Could you check a few things on this model? Use its own coordinates, in mm. A direction names the side the tool comes from. Give positions to 0.01 mm unless a question says otherwise; leave off trailing zeros. Loops run counter-clockwise (first coordinate to the right, second up) from the corner with the lowest first, then second, coordinate; pieces in that order, holes last. Notation, with made-up numbers: M -6,-12 L 37,-12 A5 cw 37,-5 Z; hole C 36,75 d10. An arc over 180 degrees is marked long. Return JSON: item names as keys, results as strings. Group by question number.
1. For pin 1 (2.5 mm diameter, centred on x = 2, y = 23.5, fed in from -Z); pin 2 (2.5 mm diameter, centred on x = 2.5, z = -56, fed in from -Y); pin 3 (5 mm diameter, centred on y = 24.5, z = -56, fed in from +X); pin 4 (5.5 mm diameter, centred on x = 2, z = -57.5, fed in from +Y), each with a flat end and sliding along its axis, tell me the tip position at first contact or that it passes through.
2. If we mould it in two halves opening along Y, with no side actions, what happens to faces 5 (the flat face through (3, -25, -52)), 6 (the flat face through (3, -20, -57)), 7 (the cylindrical face through (0.07, -0.243, 47.953)), 8 (the flat face through (0, 11.05, 60))? For each: +Y half, -Y half, draft (parallel to the pull), parting line (faces both ways), or undercut.
3. If we section it at C-C (y = 21.5): Write out the boundary of the cut face in (x, z), plus the area to 3 significant figures.
4. For faces 1 (the flat face through (3, 0, -52)), 2 (the flat face through (-1, 0, -62)), 3 (the flat face through (3, 25, -52)), 4 (the flat face through (0, -25, -57)), which set-ups out of +Z, -Z, +X, -X, +Y, -Y let a thin tool reach every point of the face, with its end or its side?
5. Please list where these lines run through material, in increasing order: line 1 (Z direction, x = 1, y = -23); line 2 (Y direction, x = -1, z = 51.5); line 3 (Z direction, x = 2.5, y = 0).
6. If we section it at B-B (z = 54.5): Write out the boundary of the cut face in (x, y).
7. If we section it at D-D (x = 3.75): Write out the boundary of the cut face in (y, z), plus the area to 3 significant figures.
8. If we section it at A-A (x = -3): Write out the boundary of the cut face in (y, z), plus the area to 3 significant figures.
```python
from build123d import *

# Parameters (mm, degrees)
F0_W     = 10
F0_H     = 124
F1_DEPTH = 30
F3_DEPTH = 10
F4_W     = 10
F4_H     = 10
F5_DEPTH = 5


with BuildPart() as f1:
    # F0 (on Front) → F1 (new body, symmetric)
    with BuildSketch(Plane.XZ):
        Rectangle(F0_W, F0_H)
    extrude(amount=F1_DEPTH, both=True)

    # F2 (on face) → F3 (cut)
    with BuildSketch(Plane.YZ.offset(5)):
        with BuildLine():
            Line((-11.05, 62), (-11.05, 59))
            ThreePointArc((-11.05, 59), (0, 47.95), (11.05, 59))
            Line((11.05, 59), (11.05, 62))
            Line((11.05, 62), (-11.05, 62))
        make_face()
    extrude(amount=-F3_DEPTH, mode=Mode.SUBTRACT)

    # F4 (on face) → F5 (cut)
    with BuildSketch(Plane.YZ.offset(5)):
        with Locations((-25, -57)):
            Rectangle(F4_W, F4_H)
        with Locations((25, -57)):
            Rectangle(F4_W, F4_H)
        with Locations((0, -57)):
            Rectangle(F4_W, F4_H)
    extrude(amount=-F5_DEPTH, mode=Mode.SUBTRACT)


solid = f1.part
```
Answer:
{
 "1": {"pin 1": "stops at z = -52", "pin 2": "stops at y = -20", "pin 3": "stops at x = 0", "pin 4": "stops at y = 30"},
 "2": {"face 5": "draft", "face 6": "-Y half", "face 7": "undercut", "face 8": "undercut"},
 "3": {"outline": "M -5,-62 L 0,-62 L 0,-52 L 5,-52 L 5,62 L -5,62 Z", "area": "1,190 mm²"},
 "4": {"face 1": "-Z, +X", "face 2": "-Z, +X, -X, +Y, -Y", "face 3": "-Z, +X, +Y", "face 4": "-Z, +X, -Y"},
 "5": {"line 1": "z = -52 to 62", "line 2": "y = -30 to -8.11, 8.11 to 30", "line 3": "z = -52 to 47.95"},
 "6": {"outline": "M -5,-30 L 5,-30 L 5,-10.09 L -5,-10.09 Z; M -5,10.09 L 5,10.09 L 5,30 L -5,30 Z"},
 "7": {"outline": "M -30,-52 L -20,-52 L -20,-62 L -5,-62 L -5,-52 L 5,-52 L 5,-62 L 20,-62 L 20,-52 L 30,-52 L 30,62 L 11.05,62 L 11.05,59 A11.05 cw -11.05,59 L -11.05,62 L -30,62 Z", "area": "6,880 mm²"},
 "8": {"outline": "M -30,-62 L 30,-62 L 30,62 L 11.05,62 L 11.05,59 A11.05 cw -11.05,59 L -11.05,62 L -30,62 Z", "area": "7,180 mm²"}
}
